Source: CAD feature listing. Evaluate the final solid. Frame: model axes, mm. Coordinates: 2 decimals unless noted, no trailing zeros. Write each loop counter-clockwise with the first axis right and the second up, starting at its lowest first coordinate (ties: lowest second). Pieces come first, ordered by that corner, then holes. Notation, with made-up numbers: M 76.25,5.25 L 127.25,5.25 A29 cw 127.25,33.25 Z; hole C 80.25,-7 d8. An arc over 180 degrees is marked long. Answer as CSV lines item,"result". Start each with the question number.
1. Contact query for a flat-ended pin moving along its axis: pin 1 Ø1 at (x, z) = (-1, 6.5) entering from +Y. Output: stop coordinate, or through.
2. Section C-C on x = -0.5. Return the cut outline in (y, z).
3. Section B-B on y = 0.75. Return the cut outline in (x, z), plus the area to 3 significant figures.
4. Line query: probe 1 along X at (y, z) = (-0.5, 4.75); probe 2 along Y at (x, z) = (-0.65, 8.25); probe 3 along X at (y, z) = (-1.2, 3). Output: solid intervals per line, ascending. Write a range as [from, to].
5. Section A-A on z = 1.25. Return the cut outline in (x, y) (1 decimal), plus the area to 3 significant figures.
```python
from build123d import *

# Parameters (mm, degrees)
F2_DEPTH = 5
F3_R     = 1.5875
F4_DEPTH = 9
F5_DEPTH = 25


with BuildPart() as f2:
    # F1 (on Front) → F2 (new body, symmetric)
    with BuildSketch(Plane.XZ):
        Polygon((1.5875, -8), (1.5875, 0), (-1.5875, 0), (-1.5875, -8), (-8.25, -8), (-8.25, -19.5), (8.25, -19.5), (8.25, -8), align=None)
    extrude(amount=F2_DEPTH, both=True)

    # F3 (on Top) → F4 (join)
    with BuildSketch(Plane.XY):
        Circle(F3_R)
    extrude(amount=F4_DEPTH)

    # F5 (cut): a face of the model
    f5_faces = [f2.faces().sort_by_distance(p)[0] for p in [
        (0, -5, -12.5989425982),
    ]]
    extrude(f5_faces, amount=-F5_DEPTH, mode=Mode.SUBTRACT)


solid = f2.part
```
Values:
1,pin 1,"y = 1.51"
2,outline,"M -1.51,0 L 1.51,0 L 1.51,9 L -1.51,9 Z"
3,outline,"M -1.4,0 L 1.4,0 L 1.4,9 L -1.4,9 Z"
3,area,"25.2 mm²"
4,probe 1,"[-1.51, 1.51]"
4,probe 2,"[-1.45, 1.45]"
4,probe 3,"[-1.04, 1.04]"
5,outline,"C 0,0 d3.2"
5,area,"7.92 mm²"
